The listing builds one solid part. Answer for the finished solid, in the listing's coordinates (mm). Face numbers are marked on the shaded views. Coordinates: 2 decimals unless noted, no trailing zeros. Write each loop counter-clockwise with the first axis right and the second up, starting at its lowest first coordinate (ties: lowest second). Pieces come first, ordered by that corner, then holes.
from build123d import *

# Parameters (mm, degrees)
SKETCH1_W      = 30
SKETCH1_H      = 20
SKETCH1_R      = 1.65
EXTRUDE1_DEPTH = 3
EXTRUDE2_DEPTH = 25
EXTRUDE3_DEPTH = 25
SKETCH5_R      = 1
SKETCH5_W      = 17.276120282
SKETCH5_H      = 25
EXTRUDE4_DEPTH = 25


with BuildPart() as part:
    # Sketch1 → Extrude1 (new body)
    with BuildSketch(Plane(origin=(0, 0, 0), x_dir=(1, 0, 0), z_dir=(0, 1, 0))):
        with Locations((0, 5)):
            Rectangle(SKETCH1_W, SKETCH1_H)
        with Locations(Location((10, 0, 0), (0, 0, 270))):
            Circle(SKETCH1_R, mode=Mode.SUBTRACT)
        with Locations(Location((-10, 0, 0), (0, 0, 270))):
            Circle(SKETCH1_R, mode=Mode.SUBTRACT)
    extrude(amount=EXTRUDE1_DEPTH)

    # Sketch3 → Extrude2 (add)
    with BuildSketch(Plane(origin=(0, 3, 0), x_dir=(1, 0, 0), z_dir=(0, 1, 0))):
        Polygon((15, 11.950319031), (15, 15), (-15, 9.517719352), (-14.462267947, 6.575155369), (-10.171425839, 7.350425006), align=None)
        Polygon((-14.462267947, 6.575155369), (-15, 9.517719352), (-15, 6.477997906), align=None)
    extrude(amount=EXTRUDE2_DEPTH)

    # Sketch4 → Extrude3 (cut)
    with BuildSketch(Plane(origin=(0, 3, 0), x_dir=(1, 0, 0), z_dir=(0, 1, 0))):
        Polygon((-15, 9.517719352), (-15, 15), (15, 15), align=None)
    extrude(amount=-EXTRUDE3_DEPTH, mode=Mode.SUBTRACT)

    # Sketch5 → Extrude4 (cut)
    with BuildSketch(Plane(origin=(-1.628525639, 0, -8.911577554), x_dir=(0.9837094537947668, 0, -0.1797657100639655), z_dir=(0.1797657100639655, 0, 0.9837094537947668))):
        with Locations((-9.26857722, 8)):
            Circle(SKETCH5_R)
        with Locations((13.23142278, 24)):
            Circle(SKETCH5_R)
        with Locations((1.901847648, 15.5)):
            Rectangle(SKETCH5_W, SKETCH5_H)
    extrude(amount=-EXTRUDE4_DEPTH, mode=Mode.SUBTRACT)


solid = part.part
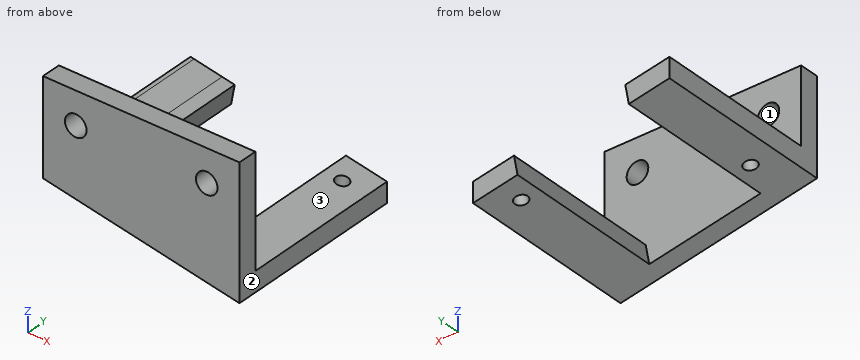
Q1. Determine the mould class of the marked faces 1, 2 and 3 for opening direction Z: released by +Z, released by -Z, zero draft, split by the parting line, or undercut.
Answers below:
face 1: undercut
face 2: zero draft
face 3: released by +Z
Q2. The part is cut by section B-B, the plane y = 25.5. Write down the section's boundary in (x, z) (3 decimals).
Answers below:
outline: (-15, -9.518) - (-8.794, -10.652) - (-8.255, -7.701) - (-10.171, -7.35) - (-15, -6.478) - close; (8.2, -13.757) - (15, -15) - (15, -11.95) - (8.74, -10.806) - close
Q3. Find the intervals of material crossed by probe 1 along X at (y, z) = (1.85, 0); probe 2 along Y at (x, z) = (4.5, -2); probe 3 along Z at (x, y) = (10, 11.75), in increasing order.
Answers below:
probe 1: x = -15 to -11.65, -8.35 to 8.35, 11.65 to 15
probe 2: y = 0 to 3
probe 3: z = -14.09 to -11.04
Q4. The part is cut by section D-D, the plane z = 3. Write down the section's boundary in (x, y).
Answers below:
outline: (-15, 0) - (15, 0) - (15, 3) - (-15, 3) - close
Q5. The part is cut by section C-C, the plane x = 3.5. Write down the section's boundary in (y, z).
Answers below:
outline: (0, -12.9) - (3, -12.9) - (3, 5) - (0, 5) - close
Q6. The part is cut by section A-A, the plane z = 0. Write down the section's boundary in (x, y).
Answers below:
outline: (-15, 0) - (-11.65, 0) - (-11.65, 3) - (-15, 3) - close; (-8.35, 0) - (8.35, 0) - (8.35, 3) - (-8.35, 3) - close; (11.65, 0) - (15, 0) - (15, 3) - (11.65, 3) - close
Q7. Given pin 1 (8 mm diameter, centred on x = -1.5, z = -9.5, fed in from +Y); pin 2 (1 mm diameter, centred on x = -11, y = 11, fed in from +Z); pin 3 (3 mm diameter, centred on y = 21.5, z = -6, fed in from -X); pin 4 (6 mm diameter, centred on x = -10, y = 20, fed in from -Z), each flat-ended and moving along its own axis, determine where each tip first touches the part or whether it passes through.
Answers below:
pin 1: stops at y = 3
pin 2: stops at z = -7.11
pin 3: stops at x = -15
pin 4: stops at z = -10.65
